Part print with two shaded views. Sizes in mm from the minimum x, y, z corner. Give positions to 0.01 mm unless a question says otherwise; leave off trailing zeros. Order: outer loops, then holes, each group sorted by start corner. A loop starts at its lowest first (then second) coordinate and runs counter-clockwise, first axis right, second up.
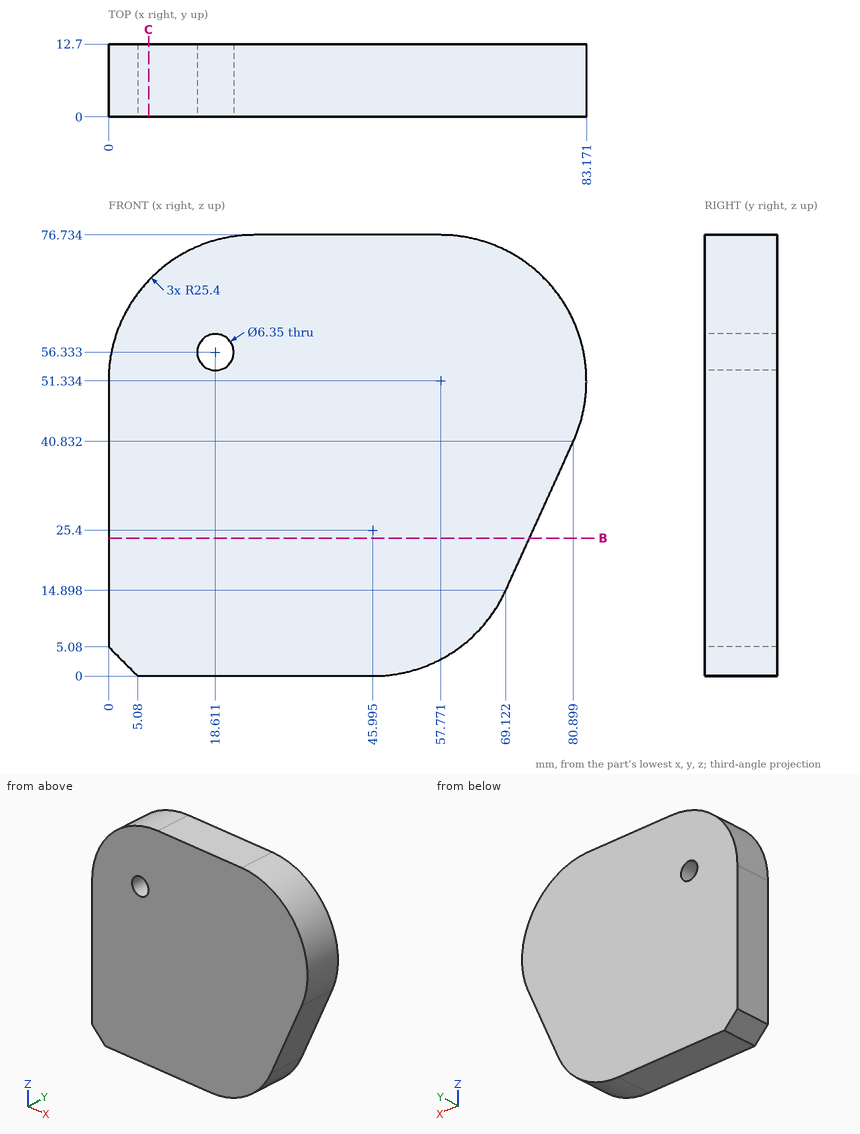
1. Pin check, flat tips, straight feed: P1, Ø5, axis at x = 16.5, y = 5, coming from the +Z side (1 decimal); P2, Ø2, axis at x = 50.5, y = 8, coming from the -Z side. Stop position of each tip, or through.
2. Saw through at B-B on z = 24. Give the cut face in (x, y) (1 decimal).
3. Saw through at C-C on x = 7. Give the cut face in (y, z) (1 decimal), plus the area to 3 significant figures.
4. Wall check: line 1 (X direction, y = 1.5, z = 57) (1 decimal); line 2 (X direction, y = 8.75, z = 56) (1 decimal); line 3 (Z direction, x = 25, y = 2). Give the ranges that are in metal, low to high.
Reported:
1. P1: stops at z = 75.9
1. P2: stops at z = 0.24
2. outline: (0, 0) - (73.3, 0) - (73.3, 12.7) - (0, 12.7) - close
3. outline: (0, 0) - (12.7, 0) - (12.7, 68.8) - (0, 68.8) - close
3. area: 874 mm2
4. line 1: x = 0.6 to 15.5, 21.7 to 82.5
4. line 2: x = 0.4 to 15.5, 21.8 to 82.7
4. line 3: z = 0 to 76.73
